Can you work these out from the drawing? Everything is in mm from the part's minimum corner. Give positions to 0.01 mm unless a question says otherwise; leave off trailing zeros. Loops run counter-clockwise (first coordinate to the right, second up) from the corner with the lowest first, then second, coordinate; pieces in that order, holes last. Notation, with made-up numbers: (79.5, 3.25) - (138.5, 3.25) arc R29 cw to (138.5, 39.25) - close; hole circle Ø2 at (-18.5, -14.75). An arc over 180 degrees is marked (long way). Answer in a Markdown table with one row per item.
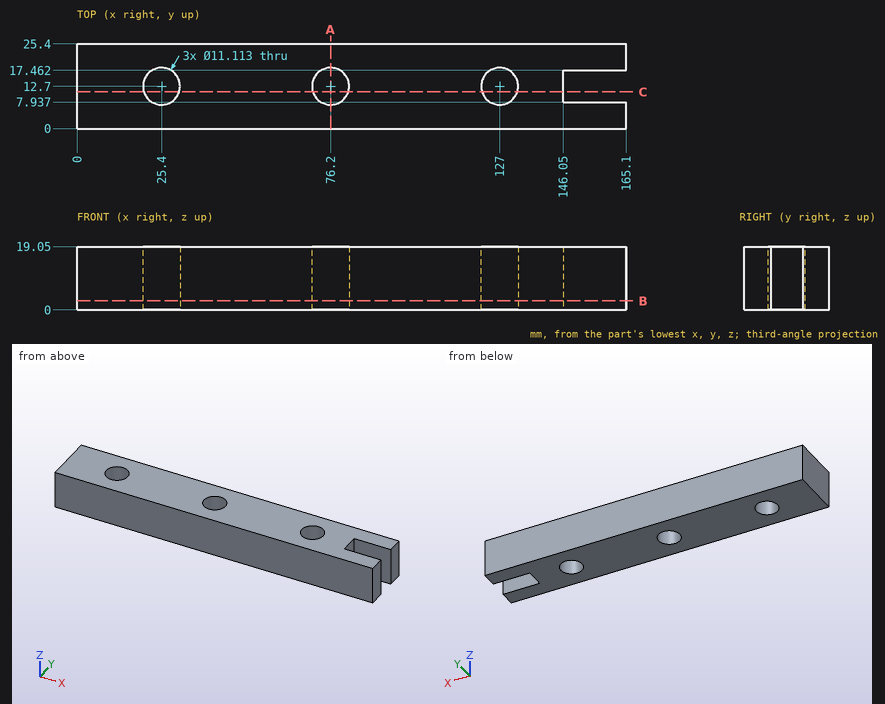
Q1. Imagine slicing it at B-B, the plane z = 2.75. Write out the boundary of the cut face in (x, y).
Checked values:
| item | result |
|---|---|
| outline | (0, 0) - (165.1, 0) - (165.1, 7.94) - (146.05, 7.94) - (146.05, 17.46) - (165.1, 17.46) - (165.1, 25.4) - (0, 25.4) - close; hole circle Ø11.11 at (25.4, 12.7); hole circle Ø11.11 at (76.2, 12.7); hole circle Ø11.11 at (127, 12.7) |
Q2. Imagine slicing it at A-A, the plane x = 76.2. Write out the boundary of the cut face in (y, z), and give its area (3 significant figures).
Checked values:
| item | result |
|---|---|
| outline | (0, 0) - (7.14, 0) - (7.14, 19.05) - (0, 19.05) - close; (18.26, 0) - (25.4, 0) - (25.4, 19.05) - (18.26, 19.05) - close |
| area | 272 mm² |
Q3. If I drill on line 1 (Y direction, x = 127, z = 6); line 2 (Y direction, x = 71.5, z = 16.75) (1 decimal), over which ranges is the centre line in solid material (lowest first)? Write a range as [from, to].
Checked values:
| item | result |
|---|---|
| line 1 | y = [0, 7.14], [18.26, 25.4] |
| line 2 | y = [0, 9.7], [15.7, 25.4] |
Q4. Imagine slicing it at C-C, the plane y = 11. Write out the boundary of the cut face in (x, z).
Checked values:
| item | result |
|---|---|
| outline | (0, 0) - (20.11, 0) - (20.11, 19.05) - (0, 19.05) - close; (30.69, 0) - (70.91, 0) - (70.91, 19.05) - (30.69, 19.05) - close; (81.49, 0) - (121.71, 0) - (121.71, 19.05) - (81.49, 19.05) - close; (132.29, 0) - (146.05, 0) - (146.05, 19.05) - (132.29, 19.05) - close |
Q5. For pin 1 (9 mm diameter, centred on x = 76.2, y = 12.7, fed in from -Z); pin 2 (3 mm diameter, centred on y = 13.5, z = 13, fed in from +X), each with a flat end and sliding along its axis, tell me the tip position at first contact or that it passes through.
Checked values:
| item | result |
|---|---|
| pin 1 | passes through |
| pin 2 | stops at x = 146.05 |
